Geometry check sheet. Reference: the model listing, model coordinates, mm. Face numbers are marked on the shaded views. Coordinates: 2 decimals unless noted, no trailing zeros. Order: outer loops, then holes, each group sorted by start corner. A loop starts at its lowest first (then second) coordinate and runs counter-clockwise, first axis right, second up.
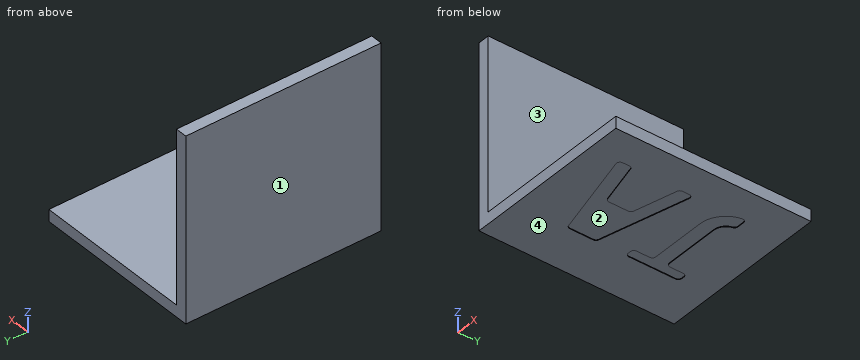
Autodesk Inventor part; units mm, degrees
ref_plane "YZ Plane" through (0, 0, 0) normal (1, 0, 0) x (0, 1, 0)
ref_plane "XZ Plane" through (0, 0, 0) normal (0, 1, 0) x (-1, 0, 0)
ref_plane "XY Plane" through (0, 0, 0) normal (0, 0, 1) x (1, 0, 0)
sketch "Sketch1" plane through (0, 0, 0) normal (0, 1, 0) x (-1, 0, 0)
  line L0 (17, 250) -> (0, 250)
  line L1 (0, 250) -> (0, 0)
  line L2 (0, 0) -> (17, 0)
  line L3 (17, 0) -> (17, 250)
  line L4 (17, 0) -> (-233, 0)
  line L5 (-233, 0) -> (-233, -17)
  line L6 (-233, -17) -> (17, -17)
  line L7 (17, -17) -> (17, 0)
  dimension "d0" = 17
  dimension "d1" = 250
  dimension "d2" = 250
extrude "Extrusion1" add sketch "Sketch1" along normal blind 284.5
sketch "Sketch2" plane through (233, 0, -17) normal (0, 0, -1) x (-1, 0, 0)
  line L0 (0, 0) -> (250, 0)
  line L1 (250, 0) -> (250, 284.5)
  line L2 (0, 284.5) -> (250, 284.5)
  line L3 (0, 0) -> (0, 284.5)
  line L4 (182.1785, 237.4156) -> (168.1785, 237.4156)
  line L5 (168.1785, 237.4156) -> (168.1785, 159.4156)
  line L6 (168.1785, 159.4156) -> (182.1785, 159.4156)
  line L7 (182.1785, 159.4156) -> (182.1785, 237.4156)
  line L8 (168.1785, 208.4156) -> (82.1785, 208.4156)
  line L9 (82.1785, 208.4156) -> (82.1785, 188.4156)
  line L10 (82.1785, 188.4156) -> (168.1785, 188.4156)
  line L11 (168.1785, 188.4156) -> (168.1785, 208.4156)
  arc A0 (64.6656, 225.9286) -> (82.1785, 208.4156) centre (82.1785, 225.9286) ccw
  line L12 (82.1785, 225.9286) -> (64.6656, 225.9286) construction
  line L13 (82.1785, 225.9286) -> (82.1785, 208.4156) construction
  arc A1 (44.6656, 225.9286) -> (82.1785, 188.4156) centre (82.1785, 225.9286) ccw
  line L14 (64.6656, 225.9286) -> (44.6656, 225.9286)
  line L15 (182.3419, 116.525) -> (46.5005, 150.394)
  line L16 (46.5005, 150.394) -> (46.5005, 130.394)
  line L17 (46.5005, 130.394) -> (114.6042, 113.4139)
  line L18 (114.6042, 113.4139) -> (114.6042, 93.4139)
  line L19 (182.3419, 116.525) -> (182.3419, 95.525)
  line L20 (133.1096, 95.525) -> (42.0362, 95.525)
  line L21 (182.3419, 74.525) -> (46.5005, 40.6559)
  line L22 (46.5005, 40.6559) -> (46.5005, 60.6559)
  line L23 (46.5005, 60.6559) -> (114.6042, 77.6361)
  line L24 (114.6042, 77.6361) -> (114.6042, 97.6361)
  line L25 (182.3419, 74.525) -> (182.3419, 95.525)
  point P0 (233, 0)
  dimension "d5" = 90
  dimension "d6" = 21
  dimension "d7" = 140
  dimension "d8" = 20
  dimension "d9" = 20
  dimension "d12" = 68.1037
  dimension "d13" = 78
  dimension "d14" = 20
  dimension "d15" = 29
  dimension "d16" = 14
  dimension "d18" = 86
  dimension "d20" = 76
extrude "Extrusion2" cut sketch "Sketch2" against normal blind 1 contours L7 L6 L5 L4 | L5 L10 L9 L8 | L9 A1 L14 A0 | L19 L25 L21 L22 L23 L24 L18 L17 L16 L15
fillet "Fillet1" radius 5 16 edges at (50.6581, 116.525, -16.5) (50.6581, 74.525, -16.5) (50.8215, 159.4156, -16.5) (64.8215, 188.4156, -16.5) (118.3958, 113.4139, -16.5) (118.3958, 77.6361, -16.5) (186.4995, 40.6559, -16.5) (186.4995, 60.6559, -16.5) (186.4995, 130.394, -16.5) (186.4995, 150.394, -16.5) (168.3344, 225.9286, -16.5) (188.3344, 225.9286, -16.5) (64.8215, 237.4156, -16.5) (50.8215, 237.4156, -16.5) (64.8215, 159.4156, -16.5) (64.8215, 208.4156, -16.5)
equation "\"d15\" = 0.5 * d13 - 0.5 * d14"
properties part number "TableroEscritoSimplificado"
Item 1: Thickness scan on line 1 along X through (y, z) = (188, 157.5); line 2 along Z through (x, y) = (114.5, 75). Record the ranges inside material, lowest first.
Item 2: Depth check by flat-ended pin: P1, Ø1, axis at x = 16, y = 99, coming from the +Z side; P2, Ø1, axis at y = 223.5, z = 64.5, coming from the +X side. Enter the tip coordinate at first touch or a pass-through.
Item 3: Release check for a two-part mould opening along X. For the marked faces 1, 2, 3 and 4 record: pulls with the +X half, pulls with the -X half, needs draft (parallel to the pull), parting line crosses it, or undercut.
Item 4: Sectioned sample at A-A (y = 261). Record the cut outline in (x, z), and give its area (3 significant figures).
Item 5: Sectioned sample at B-B (x = 97). Record the cut outline in (y, z).
Item 6: Sectioned sample at D-D (y = 196.5). Record the cut outline in (x, z), and give its area (3 significant figures).
Item 7: Sectioned sample at C-C (z = 111). Record the cut outline in (x, y), and give its area (3 significant figures).
Geometry check:
1. line 1: x = -17 to 0
1. line 2: z = -16 to 0
2. P1: stops at z = 0
2. P2: stops at x = 0
3. face 1: pulls with the -X half
3. face 2: undercut
3. face 3: pulls with the +X half
3. face 4: needs draft
4. outline: (-17, -17) - (233, -17) - (233, 0) - (0, 0) - (0, 250) - (-17, 250) - close
4. area: 8,500 mm2
5. outline: (0, -17) - (62.97, -17) - (62.97, -16) - (128.08, -16) - (128.08, -17) - (188.42, -17) - (188.42, -16) - (208.42, -16) - (208.42, -17) - (284.5, -17) - (284.5, 0) - (0, 0) - close
6. outline: (-17, -17) - (50.82, -17) - (50.82, -16) - (174.08, -16) - (174.08, -17) - (233, -17) - (233, 0) - (0, 0) - (0, 250) - (-17, 250) - close
6. area: 8,380 mm2
7. outline: (-17, 0) - (0, 0) - (0, 284.5) - (-17, 284.5) - close
7. area: 4,840 mm2
